Here's the drawing with two shaded views (mm, measured from the low corner). I have some questions. Give positions to 0.01 mm unless a question says otherwise; leave off trailing zeros. Write each loop counter-clockwise with the first axis right and the second up, starting at its lowest first coordinate (ties: lowest second). Pieces come first, ordered by that corner, then holes. Notation, with made-up numbers: (-7, 70) -> (7, 70) arc R25 ccw to (7, 89) -> close; hole circle Ø2 at (-27.5, 14.5). An arc over 180 degrees is marked (long way). One line per item, written item: value.
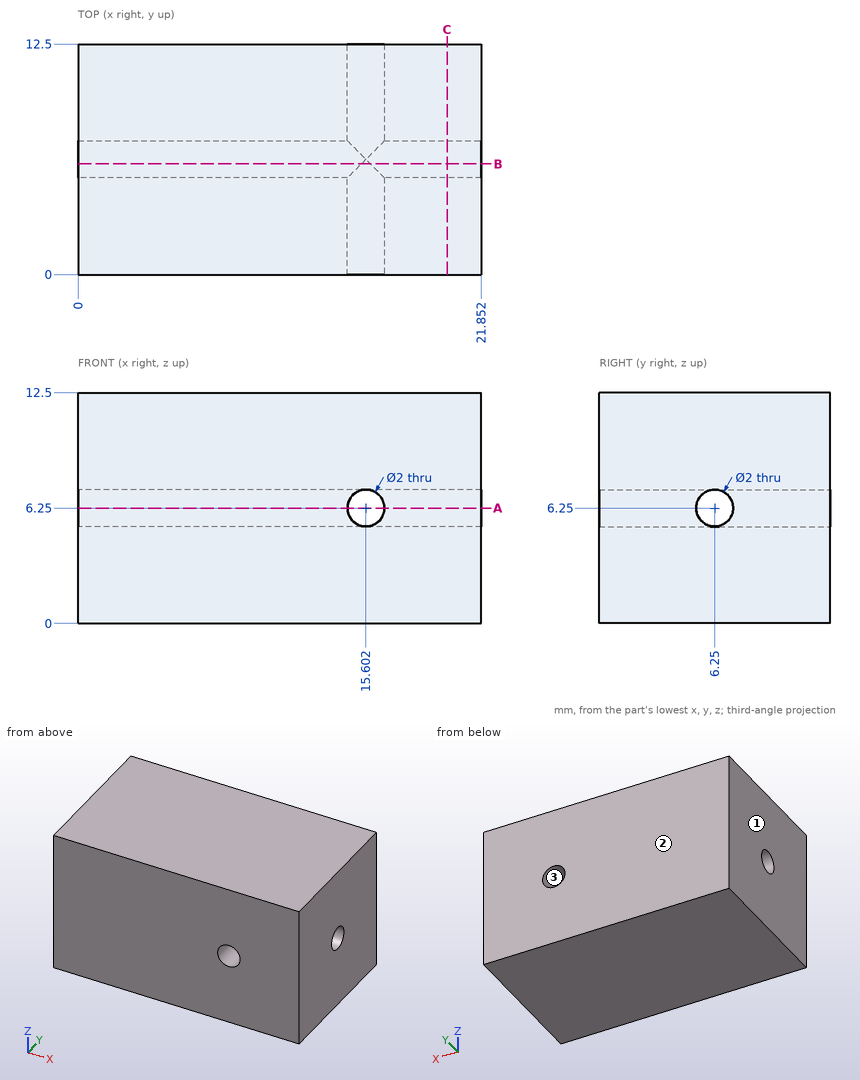
1) We'd pull the mould along X, two halves only. Please class the marked faces 1, 2 and 3: released by +X, released by -X, zero draft, split by the parting line, or undercut.
Answer list:
face 1: released by -X
face 2: zero draft
face 3: undercut
2) If we section it at C-C (x = 20): Write out the boundary of the cut face in (y, z).
Answer list:
outline: (0, 0) -> (12.5, 0) -> (12.5, 12.5) -> (0, 12.5) -> close; hole circle Ø2 at (6.25, 6.25)
3) I need wall thicknesses on L1, parallel to Z at x = 20.25, y = 6.25; L2, parallel to X at y = 4, z = 6.25. Which ranges of each line are inside material? Lowest first, please.
Answer list:
L1: z = 0 to 5.25, 7.25 to 12.5
L2: x = 0 to 14.6, 16.6 to 21.85
4) If we section it at B-B (y = 6): Write out the boundary of the cut face in (x, z).
Answer list:
outline: (0, 0) -> (21.85, 0) -> (21.85, 5.28) -> (15.85, 5.28) arc R1 cw to (15.35, 5.28) -> (0, 5.28) -> close; (0, 7.22) -> (15.35, 7.22) arc R1 cw to (15.85, 7.22) -> (21.85, 7.22) -> (21.85, 12.5) -> (0, 12.5) -> close
5) If we section it at A-A (z = 6.25): Write out the boundary of the cut face in (x, y).
Answer list:
outline: (0, 0) -> (14.6, 0) -> (14.6, 5.25) -> (0, 5.25) -> close; (0, 7.25) -> (14.6, 7.25) -> (14.6, 12.5) -> (0, 12.5) -> close; (16.6, 0) -> (21.85, 0) -> (21.85, 5.25) -> (16.6, 5.25) -> close; (16.6, 7.25) -> (21.85, 7.25) -> (21.85, 12.5) -> (16.6, 12.5) -> close
